CAD build for the part. Positions are in the model's coordinates, mm. Face numbers are marked on the shaded views. A direction names the side the tool comes from. Give positions to 0.01 mm unless a question says otherwise; leave off trailing zeros. Order: outer loops, then holes, each group sorted by start corner. A loop starts at its lowest first (then second) coordinate and runs counter-clockwise, first axis right, second up.
Item 1: Wall check: L1, parallel to X at y = 17.85, z = 65; L2, parallel to Z at x = -31, y = 1; L3, parallel to Y at x = -34.5, z = 45.5 (3 decimals). Give the ranges that are in metal, low to high.
Item 2: Two-plate mould, pull along Z, no slides. Class the marked faces 3, 4 and 5: released by +Z, released by -Z, zero draft, split by the parting line, or undercut.
Item 3: Band-saw the part on C-C on x = -37.5. Give the cut face in (y, z) (3 decimals), plus the area to 3 significant figures.
Item 4: Flat gauge pin, fed straight in: P1, Ø10, axis at x = -8.5, z = 40.5, coming from the -Y side (3 decimals). Where does the tip first touch, or does it go through?
Item 5: Band-saw the part on A-A on z = 65. Give the cut face in (x, y) (3 decimals).
Item 6: Which spindle directions (+Z, -Z, +X, -X, +Y, -Y) get a long thin tool onto all of the face, cutting with end or side? Do the marked faces 1 and 2. Say none if no direction does.
Item 7: Band-saw the part on D-D on x = -7. Give the cut face in (y, z) (3 decimals), plus the area to 3 significant figures.
Item 8: Band-saw the part on B-B on y = 6. Give the cut face in (x, z), plus the area to 3 significant figures.
```python
from build123d import *

# Parameters (mm, degrees)
BOSS_EXTRUDE1_DEPTH = 4
SKETCH2_W           = 75
SKETCH2_H           = 4
BOSS_EXTRUDE2_DEPTH = 72
BOSS_EXTRUDE3_DEPTH = 4
SKETCH5_R           = 3
CUT_EXTRUDE1_DEPTH  = 4
FILLET1_R           = 3


with BuildPart() as part:
    # Sketch1 → Boss-Extrude1 (new body)
    with BuildSketch(Plane.XY):
        with BuildLine():
            Line((0, 15.875), (0, 19.875))
            Line((0, 19.875), (-75, 19.875))
            Line((-75, 19.875), (-75, 15.875))
            Line((-75, 15.875), (-6.432235, -14.51351))
            ThreePointArc((-6.432235, -14.51351), (-15.530898, 3.287373), (0, 15.875))
        make_face()
    extrude(amount=BOSS_EXTRUDE1_DEPTH)

    # Sketch2 → Boss-Extrude2 (add)
    with BuildSketch(Plane.XY.offset(4)):
        with Locations((-37.5, 17.875)):
            Rectangle(SKETCH2_W, SKETCH2_H)
    extrude(amount=BOSS_EXTRUDE2_DEPTH)

    # Sketch4 → Boss-Extrude3 (add)
    with BuildSketch(Plane.XY.offset(76)):
        with BuildLine():
            Line((-75, 19.875), (-75, 15.875))
            Line((-75, 15.875), (-6.432235, -14.51351))
            ThreePointArc((-6.432235, -14.51351), (-15.530898, 3.287373), (0, 15.875))
            Line((0, 15.875), (0, 19.875))
            Line((0, 19.875), (-75, 19.875))
        make_face()
    extrude(amount=BOSS_EXTRUDE3_DEPTH)

    # Sketch5 → Cut-Extrude1 (cut)
    with BuildSketch(Plane(origin=(0, 19.875, 0), x_dir=(1, 0, 0), z_dir=(0, 1, 0))):
        with Locations(Location((-37.5, -15, 0), (0, 0, 270))):
            Circle(SKETCH5_R)
        with Locations(Location((-37.5, -65, 0), (0, 0, 270))):
            Circle(SKETCH5_R)
    extrude(amount=-CUT_EXTRUDE1_DEPTH, mode=Mode.SUBTRACT)

    # Fillet1
    fillet1_edges = [part.edges().sort_by_distance(p)[0] for p in [
        (-6.432235, -14.51351, 78),
        (-6.432235, -14.51351, 2),
    ]]
    fillet(fillet1_edges, radius=FILLET1_R)


solid = part.part
```
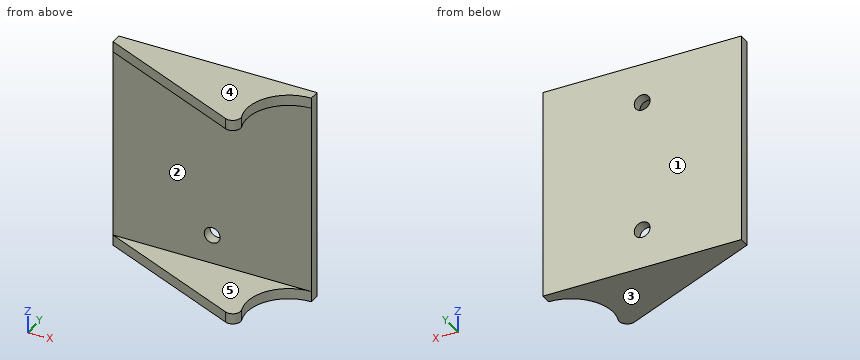
The answers:
1. L1: x = -75 to -40.5, -34.5 to 0
1. L2: z = 0 to 4, 76 to 80
1. L3: y = 15.875 to 19.875
2. face 3: released by -Z
2. face 4: released by +Z
2. face 5: undercut
3. outline: (-0.745, 0) - (19.875, 0) - (19.875, 12) - (15.875, 12) - (15.875, 4) - (-0.745, 4) - close; (-0.745, 76) - (15.875, 76) - (15.875, 68) - (19.875, 68) - (19.875, 80) - (-0.745, 80) - close; (15.875, 18) - (19.875, 18) - (19.875, 62) - (15.875, 62) - close
3. area: 405 mm2
4. P1: stops at y = 15.875
5. outline: (-75, 15.875) - (-40.5, 15.875) - (-40.5, 19.875) - (-75, 19.875) - close; (-34.5, 15.875) - (0, 15.875) - (0, 19.875) - (-34.5, 19.875) - close
6. face 1: +Z, -Z, +X, -X, +Y
6. face 2: +X, -X, -Y
7. outline: (14.248, 0) - (19.875, 0) - (19.875, 80) - (14.248, 80) - (14.248, 76) - (15.875, 76) - (15.875, 4) - (14.248, 4) - close
7. area: 333 mm2
8. outline: (-52.72, 0) - (-14.7, 0) - (-14.7, 4) - (-52.72, 4) - close; (-52.72, 76) - (-14.7, 76) - (-14.7, 80) - (-52.72, 80) - close
8. area: 304 mm2
